Here's how the part is built. I have some questions about the finished solid (model axes, mm). Coordinates: 2 decimals unless noted, no trailing zeros. Write each loop counter-clockwise with the first axis right and the second up, starting at its lowest first coordinate (ties: lowest second). Pieces come first, ordered by that corner, then holes.
(1) Imagine slicing it at D-D, the plane x = 25. List the corners of the cut face in (y, z) for me, plus the area to 3 significant figures.
(2) Imagine slicing it at A-A, the plane z = -13.5. List the corners of the cut face in (x, y) for me, plus the area to 3 significant figures.
(3) Thinking about a two-plate mould opening in Z: for faces 1 (the flat face through (90, 1, -22)), 2 (the cylindrical face through (44.5, 1.48, -13.43)), 3 (the cylindrical face through (87.9, 1.5, -42)), which applies, released by +Z, released by -Z, zero draft, split by the parting line, or undercut?
(4) Please list where these lines run through material, in increasing order: probe 1 along Z at (x, y) = (46, 1.9); probe 2 along Z at (x, y) = (25, 1.35); probe 3 along X at (y, z) = (2.4, -30.5).
(5) For pin 1 Ø1 at (y, z) = (2, -27.5) entering from -X, with a flat end and sliding along its axis, tell me the tip position at first contact or that it passes through.
(6) Imagine slicing it at C-C, the plane x = 46. List the corners of the cut face in (y, z) for me, plus the area to 3 significant figures.
(7) Imagine slicing it at B-B, the plane y = 1.3. List the corners of the cut face in (x, z) for me, plus the area to 3 significant figures.
Autodesk Fusion 360 part; units mm, degrees
sketch "Sketch1" plane through (0, 0, 0) normal (0, 1, 0) x (1, 0, 0)
  line L0 (7, 0) -> (83, 0)
  line L1 (90, 7) -> (90, 37)
  line L2 (83, 44) -> (7, 44)
  line L3 (0, 37) -> (0, 7)
  line L4 (0, 22) -> (90, 22) construction
  circle A0 centre (25, 22) radius 3.5
  circle A1 centre (25, 22) radius 32.5 construction
  arc A2 (7, 44) -> (0, 37) centre (7, 37) ccw
  arc A3 (90, 37) -> (83, 44) centre (83, 37) ccw
  arc A4 (0, 7) -> (7, 0) centre (7, 7) ccw
  arc A5 (83, 0) -> (90, 7) centre (83, 7) ccw
  line L5 (46, 63.3038) -> (46, -13) construction
  circle A6 centre (46, 30.5) radius 1.5
  circle A7 centre (46, 13.5) radius 1.5
  point P0 (90, 0)
  point P1 (0, 44)
  dimension "szerokosc" = 90
  dimension "wysokosc" = 44
  dimension "d_osi" = 7
  dimension "d4" = 25
  dimension "d_kola" = 65
  dimension "d6" = 7
  dimension "d7" = 7
  dimension "d8" = 7
  dimension "d9" = 7
  dimension "d10" = 3
  dimension "d11" = 3
  dimension "miedzy_otworami" = 17
  dimension "d13" = 8.5
  dimension "d14" = 21
extrude "Extrude1" add sketch "Sketch1" along normal blind 3
sketch "Sketch2" plane through (0, 3, 0) normal (0, 1, 0) x (-1, 0, 0)
  circle A0 centre (-25, -22) radius 3.5
  circle A1 centre (-46, -30.5) radius 1.5
  circle A2 centre (-46, -13.5) radius 1.5
  arc A3 (-83, 0) -> (-90, -7) centre (-83, -7) ccw
  line L0 (-90, -7) -> (-90, -37)
  arc A4 (-90, -37) -> (-83, -44) centre (-83, -37) ccw
  line L1 (-83, -44) -> (-7, -44)
  arc A5 (-7, -44) -> (0, -37) centre (-7, -37) ccw
  line L2 (0, -37) -> (0, -7)
  arc A6 (0, -7) -> (-7, 0) centre (-7, -7) ccw
  line L3 (-7, 0) -> (-83, 0)
equation "wysokosc = szerokosc / 3 + 2 * d_osi"
equation "d6 = d_osi"
equation "d7 = d_osi"
equation "d8 = d_osi"
equation "d9 = d_osi"
equation "miedzy_otworami = 20 mm - 3 mm"
equation "d13 = miedzy_otworami / 2"
Recorded:
1. outline: (0, -44) - (3, -44) - (3, -25.5) - (0, -25.5) - close; (0, -18.5) - (3, -18.5) - (3, 0) - (0, 0) - close
1. area: 111 mm2
2. outline: (0, 0) - (44.5, 0) - (44.5, 3) - (0, 3) - close; (47.5, 0) - (90, 0) - (90, 3) - (47.5, 3) - close
2. area: 261 mm2
3. face 1: zero draft
3. face 2: undercut
3. face 3: released by -Z
4. probe 1: z = -44 to -32, -29 to -15, -12 to 0
4. probe 2: z = -44 to -25.5, -18.5 to 0
4. probe 3: x = 0 to 44.5, 47.5 to 90
5. pin 1: stops at x = 0
6. outline: (0, -44) - (3, -44) - (3, -32) - (0, -32) - close; (0, -29) - (3, -29) - (3, -15) - (0, -15) - close; (0, -12) - (3, -12) - (3, 0) - (0, 0) - close
6. area: 114 mm2
7. outline: (0, -37) arc R7 ccw to (7, -44) - (83, -44) arc R7 ccw to (90, -37) - (90, -7) arc R7 ccw to (83, 0) - (7, 0) arc R7 ccw to (0, -7) - close; hole circle Ø7 at (25, -22); hole circle Ø3 at (46, -30.5); hole circle Ø3 at (46, -13.5)
7. area: 3,870 mm2
